The listing builds one solid part. Answer for the finished solid, in the listing's coordinates (mm). A direction names the side the tool comes from. Round coordinates to 2 decimals unless told otherwise and drop trailing zeros. Write each loop counter-clockwise with the first axis right and the second up, starting at its lowest first coordinate (ties: lowest second). Pieces come first, ordered by that corner, then holes.
(1) Each of these flat-tipped pins is pushed along its axis until it touches: pin 1 Ø1.2 at (x, y) = (-1, 1) entering from +Z; pin 2 Ø3 at (y, z) = (5.5, 4.5) entering from +X; pin 3 Ø1 at (y, z) = (1, -5) entering from +X. Where does it stop, or does it pass through?
(2) For faces 1 (the face through (5, 0, 7)), 2 (the face through (0, 4.2, 3.5)), determine the directions among +Z, -Z, +X, -X, +Y, -Y from which every point of the face is accessible in a straight line to the end or side of a thin tool.
(3) Find the intervals of material crossed by probe 1 along Z at (x, y) = (-7, 1.5); probe 2 along Z at (x, y) = (0.25, 1.5); probe 3 along Y at (x, z) = (-6.75, 3.5), in increasing order.
(4) The mould has two halves that part along Y. Classify faces 3 (the face through (0, 0, -20)), 4 (the face through (-1.73, -7.81, 3.56)), 5 (the face through (-1.97, 3.48, 4.89)), 6 (the face through (-3.6, -2.1, 3.5)): +Y half, -Y half, draft (parallel to the pull), parting line (faces both ways), or undercut.
(5) A cutting plane is placed at A-A, the plane z = -15. Give the vertices of the cut face in (x, y), and give its area (3 significant figures).
from build123d import *

# Parameters (mm, degrees)
SKETCH1_W          = 20
SKETCH1_H          = 6
SKETCH4_R          = 8
EXTRUDE1_DEPTH     = 7
FILLET1_R          = 0.48
CHAMFER1_SIZE      = 0.48
CHAMFER1_SIZE2     = 0.277128129
CUT_EXTRUDE1_DEPTH = 3.5
SKETCH7_R          = 4.618802154
CUT_EXTRUDE4_DEPTH = 3.5
CUT_EXTRUDE4_DRAFT = -45
SKETCH8_R          = 4
CUT_EXTRUDE5_DEPTH = 1.166666667
CUT_EXTRUDE5_DRAFT = -60


with BuildPart() as part:
    # Sketch1 → Revolve1 (revolve)
    with BuildSketch(Plane(origin=(0, 0, 0), x_dir=(0, 0, -1), z_dir=(1, 0, 0))):
        with Locations((10, 3)):
            Rectangle(SKETCH1_W, SKETCH1_H)
    revolve(axis=Axis((0, 0, 0), (0, 0, 1)))

    # Sketch4 → Extrude1 (add)
    with BuildSketch(Plane.XY):
        Circle(SKETCH4_R)
    extrude(amount=EXTRUDE1_DEPTH)

    # Fillet1
    fillet1_edges = [part.edges().sort_by_distance(p)[0] for p in [
        (-8, 0, 0),
    ]]
    fillet(fillet1_edges, radius=FILLET1_R)

    # Chamfer1
    chamfer1_edges = [part.edges().sort_by_distance(p)[0] for p in [
        (-8, 0, 7),
    ]]
    chamfer1_side = [part.faces().sort_by_distance(p)[0] for p in [
        (0, 0, 7),
    ]]
    chamfer(chamfer1_edges, length=CHAMFER1_SIZE, length2=CHAMFER1_SIZE2, reference=chamfer1_side[0])

    # Sketch6 → Cut-Extrude1 (cut)
    with BuildSketch(Plane.XY.offset(7)):
        Polygon((0, -4.618802154), (4, -2.309401077), (4, 2.309401077), (0, 4.618802154), (-4, 2.309401077), (-4, -2.309401077), align=None)
    extrude(amount=-CUT_EXTRUDE1_DEPTH, mode=Mode.SUBTRACT)


with BuildPart() as cut_extrude4_tool:
    # Sketch7 → Cut-Extrude4 (with draft: the straight prism first)
    with BuildSketch(Plane.XY.offset(7)):
        Circle(SKETCH7_R)
    extrude(amount=-CUT_EXTRUDE4_DEPTH)
    # Cut-Extrude4: the draft: its side faces are tilted about the plane it starts from
    cut_extrude4_sides = [cut_extrude4_tool.faces().sort_by_distance(p)[0] for p in [
        (-4.618802154, 0, 5.25),
    ]]
    draft(cut_extrude4_sides, Plane.XY.offset(7), CUT_EXTRUDE4_DRAFT)


with BuildPart() as part_1:
    add(part.part)

    # Cut-Extrude4: cut by cut_extrude4_tool
    add(cut_extrude4_tool.part, mode=Mode.SUBTRACT)


with BuildPart() as cut_extrude5_tool:
    # Sketch8 → Cut-Extrude5 (with draft: the straight prism first)
    with BuildSketch(Plane.XY.offset(3.5)):
        Circle(SKETCH8_R)
    extrude(amount=-CUT_EXTRUDE5_DEPTH)
    # Cut-Extrude5: the draft: its side faces are tilted about the plane it starts from
    cut_extrude5_sides = [cut_extrude5_tool.faces().sort_by_distance(p)[0] for p in [
        (-4, 0, 2.916666667),
    ]]
    draft(cut_extrude5_sides, Plane.XY.offset(3.5), CUT_EXTRUDE5_DRAFT)


with BuildPart() as part_2:
    add(part_1.part)

    # Cut-Extrude5: cut by cut_extrude5_tool
    add(cut_extrude5_tool.part, mode=Mode.SUBTRACT)


solid = part_2.part
Solutions:
1. pin 1: stops at z = 2.35
1. pin 2: stops at x = 6.93
1. pin 3: stops at x = 5.98
2. face 1: +Z, +X, -X, +Y, -Y
2. face 2: +Z
3. probe 1: z = 0 to 7
3. probe 2: z = -20 to 2.33
3. probe 3: y = -4.29 to 4.29
4. face 3: draft
4. face 4: parting line
4. face 5: undercut
4. face 6: undercut
5. outline: circle Ø12 at (0, 0)
5. area: 113 mm2
